The model under review builds one solid part; all positions refer to its coordinate system, in mm. Coordinates: 2 decimals unless noted, no trailing zeros. Write each loop counter-clockwise with the first axis right and the second up, starting at its lowest first coordinate (ties: lowest second). Pieces come first, ordered by that corner, then holes.
1) Add section A-A, the plane x = 754. State the section outline as (y, z) points, then the cut area to 3 significant figures.
2) For P1, Ø10, axis at x = 95.5, y = 107, coming from the +Z side; P2, Ø2, axis at x = 438.5, y = 66.5, coming from the +Z side (3 decimals); P3, Ø1.5, axis at x = 393, y = 28.5, coming from the +Z side, all flat-tipped, find the tip position at first contact; note any pin that passes through.
3) Add section C-C, the plane y = 76.5. State the section outline as (x, z) points (3 decimals).
4) For line 1 (Z direction, x = 307.5, y = 141); line 2 (Z direction, x = 213, y = 14), list the stretches that pass through material, from the lowest coordinate up.
5) Add section B-B, the plane y = 15. State the section outline as (x, z) points (3 decimals), then the cut area to 3 significant figures.
Autodesk Inventor part; units mm, degrees
ref_plane "YZ Plane" through (0, 0, 0) normal (1, 0, 0) x (0, 1, 0)
ref_plane "XZ Plane" through (0, 0, 0) normal (0, 1, 0) x (-1, 0, 0)
ref_plane "XY Plane" through (0, 0, 0) normal (0, 0, 1) x (1, 0, 0)
sketch "Profile" plane through (0, 0, 0) normal (0, 0, 1) x (1, 0, 0)
  line L0 (0, 0) -> (0, 330.2)
  line L1 (0, 0) -> (152.4, 0)
  line L2 (152.4, 0) -> (152.4, 342.9)
  line L3 (152.4, 342.9) -> (139.7, 342.9) construction
  line L4 (152.4, 342.9) -> (139.7, 342.9) construction
  arc A0 (152.4, 342.9) -> (137.4098, 355.3918) centre (139.7, 342.9) ccw
  line L5 (0, 330.2) -> (137.4098, 355.3918)
  dimension "d0" = 330.2
  dimension "d1" = 152.4
  dimension "d2" = 342.9
  dimension "d3" = 12.7
  dimension "d4" = 12.7
sketch "Sketch1" plane through (0, 0, 0) normal (1, 0, 0) x (0, 1, 0)
  line L0 (0, 0) -> (0, 330.2)
  line L1 (0, 0) -> (152.4, 0)
  line L2 (152.4, 0) -> (152.4, 342.9)
  line L3 (152.4, 342.9) -> (139.7, 342.9) construction
  line L4 (152.4, 342.9) -> (139.7, 342.9) construction
  arc A0 (152.4, 342.9) -> (137.4098, 355.3918) centre (139.7, 342.9) ccw
  line L5 (0, 330.2) -> (137.4098, 355.3918)
extrude "Extrusion1" add sketch "Sketch1" along normal blind 898.525
properties part number "L" material "Granite, Cut, Polished"
Geometry results:
1. outline: (0, 0) - (152.4, 0) - (152.4, 342.9) arc R12.7 ccw to (137.41, 355.39) - (0, 330.2) - close
1. area: 52,400 mm2
2. P1: stops at z = 350.73
2. P2: stops at z = 342.575
2. P3: stops at z = 335.56
3. outline: (0, 0) - (898.525, 0) - (898.525, 344.225) - (0, 344.225) - close
4. line 1: z = 0 to 355.53
4. line 2: z = 0 to 332.77
5. outline: (0, 0) - (898.525, 0) - (898.525, 332.95) - (0, 332.95) - close
5. area: 299,000 mm2
